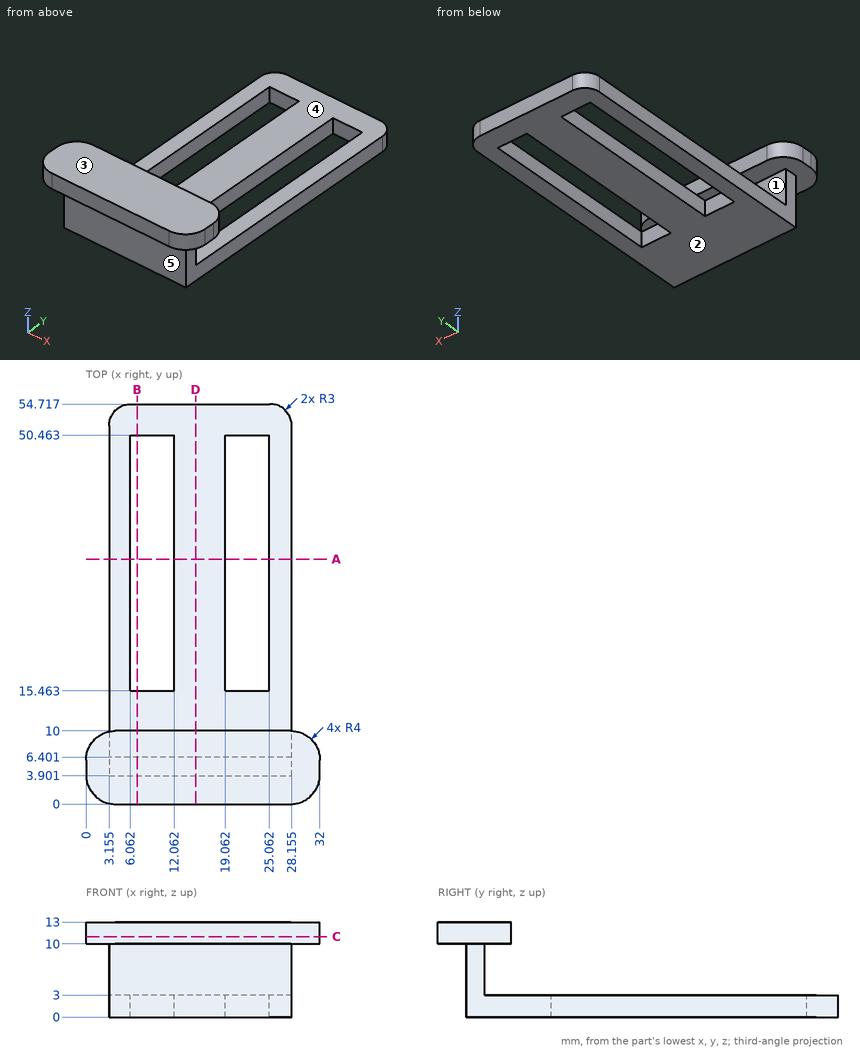
Drawing for the job (mm, zero at the part's lowest x, y, z). A direction names the side the tool comes from. Round coordinates to 2 decimals unless told otherwise and drop trailing zeros. Loops run counter-clockwise (first coordinate to the right, second up) from the corner with the lowest first, then second, coordinate; pieces in that order, holes last. Notation, with made-up numbers: (66, -34) -> (110, -34) arc R14 cw to (110, -11) -> close; hole circle Ø11 at (17.5, -11). An arc over 180 degrees is marked (long way). Answer in a Markdown table with one row per item.
Item 1: Mould opens along Z. For the marked faces 3, 4 and 5 say: +Z half, -Z half, draft (parallel to the pull), parting line (faces both ways), or undercut.
Answers below:
| item | result |
|---|---|
| face 3 | +Z half |
| face 4 | undercut |
| face 5 | draft |
Item 2: Saw through at D-D (x = 15). Write the cut outline in (y, z).
Answers below:
| item | result |
|---|---|
| outline | (0, 10) -> (3.9, 10) -> (3.9, 0) -> (54.72, 0) -> (54.72, 3) -> (6.4, 3) -> (6.4, 10) -> (10, 10) -> (10, 13) -> (0, 13) -> close |
Item 3: Pin check, flat tips, straight feed: pin 1 (3.5 mm diameter, centred on x = 15, z = 7, fed in from +Y); pin 2 (0.9 mm diameter, centred on y = 38, z = 1, fed in from -X) (1 decimal); pin 3 (3.5 mm diameter, centred on y = 33.5, z = 1, fed in from +X) (1 decimal); pin 4 (3 mm diameter, centred on x = 5.5, z = 9, fed in from -Y). Stop position of each tip, or through.
Answers below:
| item | result |
|---|---|
| pin 1 | stops at y = 6.4 |
| pin 2 | stops at x = 3.2 |
| pin 3 | stops at x = 28.2 |
| pin 4 | stops at y = 0 |
Item 4: Which spindle directions (+Z, -Z, +X, -X, +Y, -Y) get a long thin tool onto all of the face, cutting with end or side? Do the marked faces 1 and 2. Say none if no direction does.
Answers below:
| item | result |
|---|---|
| face 1 | +X, -X, +Y |
| face 2 | -Z, +X, -X, +Y, -Y |
Item 5: Saw through at B-B (x = 7). Write the cut outline in (y, z).
Answers below:
| item | result |
|---|---|
| outline | (0, 10) -> (3.9, 10) -> (3.9, 0) -> (15.46, 0) -> (15.46, 3) -> (6.4, 3) -> (6.4, 10) -> (10, 10) -> (10, 13) -> (0, 13) -> close; (50.46, 0) -> (54.72, 0) -> (54.72, 3) -> (50.46, 3) -> close |
Item 6: Saw through at C-C (z = 11). Write the cut outline in (x, y), and give its area (3 significant figures).
Answers below:
| item | result |
|---|---|
| outline | (0, 4) arc R4 ccw to (4, 0) -> (28, 0) arc R4 ccw to (32, 4) -> (32, 6) arc R4 ccw to (28, 10) -> (4, 10) arc R4 ccw to (0, 6) -> close |
| area | 306 mm² |
Item 7: Drill centre lines: L1, parallel to Y at x = 10, z = 1.75; L2, parallel to Z at x = 16, y = 32; L3, parallel to Y at x = 18, z = 11. Where is each one in solid material? Low to high. Write a range as [from, to].
Answers below:
| item | result |
|---|---|
| L1 | y = [3.9, 15.46], [50.46, 54.72] |
| L2 | z = [0, 3] |
| L3 | y = [0, 10] |
Item 8: Saw through at A-A (y = 33.5). Write the cut outline in (x, z) (1 decimal).
Answers below:
| item | result |
|---|---|
| outline | (3.2, 0) -> (6.1, 0) -> (6.1, 3) -> (3.2, 3) -> close; (12.1, 0) -> (19.1, 0) -> (19.1, 3) -> (12.1, 3) -> close; (25.1, 0) -> (28.2, 0) -> (28.2, 3) -> (25.1, 3) -> close |
